Read the model definition and answer for the solid it produces. Units are mm, in the model's axes. A direction names the side the tool comes from. Round coordinates to 2 decimals unless told otherwise and drop trailing zeros. Order: outer loops, then holes, each group sorted by start corner. A loop starts at its lowest first (then second) coordinate and runs counter-clockwise, first axis right, second up. Notation, with made-up numbers: M 80,59 L 85,59 A15 ccw 85,69 Z; hole C 23.5,29 d7. An arc over 180 degrees is marked long. Use one line per item in the form item = value. Start each with the question number.
from build123d import *

# Parameters (mm, degrees)
SALIENTE_EXTRUIR1_DEPTH = 3


with BuildPart() as part:
    # Croquis1 → Saliente-Extruir1 (new body)
    with BuildSketch(Plane.XY):
        with BuildLine():
            Line((-10, -2.5), (-10, 9.5))
            ThreePointArc((-10, 9.5), (-7.656854249, 15.156854249), (-2, 17.5))
            Line((-2, 17.5), (2, 17.5))
            ThreePointArc((2, 17.5), (7.656854249, 15.156854249), (10, 9.5))
            Line((10, 9.5), (10, -2.5))
            Line((10, -2.5), (15, -2.5))
            Line((15, -2.5), (15, -14.5))
            Line((15, -14.5), (10, -14.5))
            Line((10, -14.5), (10, -17.5))
            Line((10, -17.5), (-10, -17.5))
            Line((-10, -17.5), (-10, -14.5))
            Line((-10, -14.5), (-15, -14.5))
            Line((-15, -14.5), (-15, -2.5))
            Line((-15, -2.5), (-10, -2.5))
        make_face()
    extrude(amount=SALIENTE_EXTRUIR1_DEPTH)


solid = part.part
Item 1: Given P1, Ø1.5, axis at x = 13.5, z = 2, coming from the -Y side; P2, Ø1.5, axis at y = 1.5, z = 1, coming from the -X side; P3, Ø1.5, axis at y = 5.5, z = 1.5, coming from the +X side, each flat-ended and moving along its own axis, determine where each tip first touches the part or whether it passes through.
Item 2: A tool of negligible diameter and unlimited length cuts with its end or side. For faces 1 (the flat face through (-12, -14.5, 1)), 2 (the flat face through (12, -2.5, 1)), 3 (the flat face through (-13, -2.5, 1)), from which of +Z, -Z, +X, -X, +Y, -Y can it reach the whole face along a straight path? Write none if from no direction.
Item 3: Section A-A (z = 2.25) is taken. Write down the section's boundary in (x, y).
Item 4: Section B-B (y = 2.5) is taken. Write down the section's boundary in (x, z), and give its area (3 significant figures).
Item 5: Find the intervals of material crossed by L1, parallel to X at y = -1.5, z = 0.15; L2, parallel to Y at x = 11, z = 2.75; L3, parallel to X at y = 13, z = 0.3, in increasing order. Write a range as [from, to].
Item 6: Section C-C (x = -10.5) is taken. Write down the section's boundary in (y, z), and give its area (3 significant figures).
The answers:
q1.P1 = -14.5
q1.P2 = -10
q1.P3 = 10
q2.face_1 = +Z, -Z, -X, -Y
q2.face_2 = +Z, -Z, +X, +Y
q2.face_3 = +Z, -Z, -X, +Y
q3.outline = M -15,-14.5 L -10,-14.5 L -10,-17.5 L 10,-17.5 L 10,-14.5 L 15,-14.5 L 15,-2.5 L 10,-2.5 L 10,9.5 A8 ccw 2,17.5 L -2,17.5 A8 ccw -10,9.5 L -10,-2.5 L -15,-2.5 Z
q4.outline = M -10,0 L 10,0 L 10,3 L -10,3 Z
q4.area = 60.0 mm²
q5.L1 = [-10, 10]
q5.L2 = [-14.5, -2.5]
q5.L3 = [-9.19, 9.19]
q6.outline = M -14.5,0 L -2.5,0 L -2.5,3 L -14.5,3 Z
q6.area = 36.0 mm²
